For this review, take the finished solid that the model builds, in its own axes (mm). A direction names the side the tool comes from. Give positions to 0.01 mm unless a question says otherwise; leave off trailing zeros. Order: outer loops, then holes, each group sorted by start corner. A loop starts at its lowest first (then second) coordinate and runs counter-clockwise, first axis right, second up. Notation, with made-up numbers: (-37, 35.5) -> (-28, 35.5) arc R27 ccw to (-28, 60.5) -> close; hole circle Ø9 at (43.5, 42). An arc over 180 degrees is marked (long way). Return JSON: item names as keys, results as strings. Group by question number.
1) The part is to be moulded in two halves that separate along Y. For faces 1 (the face through (-1.08, -4.88, 7.4)), 2 (the face through (18, -100, 7)), 3 (the face through (20, -51, 7)), say which applies: released by +Y, released by -Y, zero draft, split by the parting line, or undercut.
2) To check wall thickness, follow line 1 along Y through (x, z) = (0, 5.75); line 2 along Y through (x, z) = (0, 8); line 3 along Z through (x, y) = (11.5, -82.5). State the ranges of each line that lie inside material, in increasing order.
3) For faces 4 (the face through (0, 20, 7)), 5 (the face through (15.506, -96.599, 2.265)), 6 (the face through (15.875, -94, 11)), list the 3-axis set-ups (+Z, -Z, +X, -X, +Y, -Y) from which the entire face can be reached by the end or side of a thin tool; tool diameter is ignored.
4) Add section B-B (x = -9.5). Give the boundary of the cut face in (y, z).
5) Add section A-A (x = 0). Give the boundary of the cut face in (y, z), then the cut area to 3 significant figures.
6) Insertion check: P1, Ø3, axis at x = -4, y = -55.5, coming from the +Z side; P2, Ø4, axis at x = -0.5, z = 3.5, coming from the -Y side; P3, Ø8, axis at x = 3, z = 13.5, coming from the +Y side. Each pin has a flat end and moves straight along its axis. Give the tip position at first contact, or say it passes through.
from build123d import *

# Parameters (mm, degrees)
SKETCH1_R           = 5
BOSS_EXTRUDE1_DEPTH = 15
SKETCH2_R           = 15.875
CUT_EXTRUDE1_DEPTH  = 64
SKETCH4_W           = 31.75
SKETCH4_H           = 8.5
CUT_EXTRUDE2_DEPTH  = 61


with BuildPart() as part:
    # Sketch1 → Boss-Extrude1 (new body)
    with BuildSketch(Plane.XY):
        with BuildLine():
            Line((-20, 0), (-20, -100))
            Line((-20, -100), (-15.875, -100))
            ThreePointArc((-15.875, -100), (0, -84.125), (15.875, -100))
            Line((15.875, -100), (20, -100))
            Line((20, -100), (20, 0))
            ThreePointArc((20, 0), (0, 20), (-20, 0))
        make_face()
        Circle(SKETCH1_R, mode=Mode.SUBTRACT)
    extrude(amount=BOSS_EXTRUDE1_DEPTH)

    # Sketch2 → Cut-Extrude1 (cut)
    with BuildSketch(Plane(origin=(0, -77.959645174, -41.451878628), x_dir=(1, 0, 0), z_dir=(0, 0.8829475928589248, 0.46947156278589486))):
        with Locations((0, -52.738509112)):
            Circle(SKETCH2_R)
    extrude(amount=CUT_EXTRUDE1_DEPTH, mode=Mode.SUBTRACT)

    # Sketch4 → Cut-Extrude2 (cut)
    with BuildSketch(Plane(origin=(0, -77.959645174, -41.451878628), x_dir=(1, 0, 0), z_dir=(0, 0.8829475928589248, 0.46947156278589486))):
        with Locations((0, -55.941370171)):
            Rectangle(SKETCH4_W, SKETCH4_H)
    extrude(amount=CUT_EXTRUDE2_DEPTH, mode=Mode.SUBTRACT)


solid = part.part
Evaluation:
{
 "1": {"face 1": "undercut", "face 2": "released by -Y", "face 3": "zero draft"},
 "2": {"line 1": "-67.71 to -5, 5 to 20", "line 2": "-63.48 to -5, 5 to 20", "line 3": "0 to 3.47"},
 "3": {"face 4": "+Z, -Z, +Y", "face 5": "+Z, -Z, -Y", "face 6": "+Z, -Y"},
 "4": {"outline": "(-85.24, 0) -> (17.6, 0) -> (17.6, 15) -> (-57.03, 15) -> close"},
 "5": {"outline": "(-78.52, 0) -> (-5, 0) -> (-5, 15) -> (-50.31, 15) -> close; (5, 0) -> (20, 0) -> (20, 15) -> (5, 15) -> close", "area": "1,120 mm^2"},
 "6": {"P1": "z = 13.76", "P2": "y = -75.72", "P3": "y = 20"}
}
